```python
from build123d import *

# Parameters (mm, degrees)
SKETCH5_R               = 9.525
BOSS_EXTRUDE1_DEPTH     = 15.24
SKETCH6_R               = 12.7
BOSS_EXTRUDE2_DEPTH     = 2.54
CUT_EXTRUDE1_DEPTH      = 26.272680903
CUT_EXTRUDE3_DEPTH      = 26.272680903
CUT_EXTRUDE3_DEPTH_BACK = 26.272680903
SKETCH8_R               = 1.7526
CUT_EXTRUDE4_DEPTH      = 26.272680973
CUT_EXTRUDE4_DEPTH_BACK = 26.272680973
SKETCH9_R               = 1.7526


with BuildPart() as part:
    # Sketch5 → Boss-Extrude1 (new body)
    with BuildSketch(Plane.XY):
        with Locations(Location((0, 0, 0), (0, 0, 180))):
            Circle(SKETCH5_R)
    extrude(amount=BOSS_EXTRUDE1_DEPTH)

    # Sketch6 → Boss-Extrude2 (add)
    with BuildSketch(Plane.XY.offset(15.24)):
        Circle(SKETCH6_R)
    extrude(amount=BOSS_EXTRUDE2_DEPTH)

    # Sketch7 → Cut-Extrude1 (cut, through all)
    with BuildSketch(Plane(origin=(0, 0, 0), x_dir=(-1, 0, 0), z_dir=(0, 0, -1))):
        with BuildLine():
            ThreePointArc((4.181770846, 5.456960429), (3.437499983, 5.953924622), (2.634980936, 6.35))
            Line((2.634980936, 6.35), (-2.634980936, 6.35))
            ThreePointArc((-2.634980936, 6.35), (-3.437499983, 5.953924622), (-4.181770846, 5.456960429))
            Line((-4.181770846, 5.456960429), (-6.816751782, 0.893039571))
            ThreePointArc((-6.816751782, 0.893039571), (-6.874999966, 0), (-6.816751782, -0.893039571))
            Line((-6.816751782, -0.893039571), (-4.181770846, -5.456960429))
            ThreePointArc((-4.181770846, -5.456960429), (-3.437499983, -5.953924622), (-2.634980936, -6.35))
            Line((-2.634980936, -6.35), (2.634980936, -6.35))
            ThreePointArc((2.634980936, -6.35), (3.437499983, -5.953924622), (4.181770846, -5.456960429))
            Line((4.181770846, -5.456960429), (6.816751782, -0.893039571))
            ThreePointArc((6.816751782, -0.893039571), (6.860422465, -0.447468582), (6.874999966, 0))
            ThreePointArc((6.874999966, 0), (6.860422465, 0.447468582), (6.816751782, 0.893039571))
            Line((6.816751782, 0.893039571), (4.181770846, 5.456960429))
        make_face()
    extrude(amount=-CUT_EXTRUDE1_DEPTH, mode=Mode.SUBTRACT)

    # Sketch8 → Cut-Extrude3 (cut, two sides: drawn at the far end of the back side and taken through both)
    with BuildSketch(Plane(origin=(0, 0, 0), x_dir=(0, 0, -1), z_dir=(1, 0, 0)).offset(-CUT_EXTRUDE3_DEPTH_BACK)):
        with Locations((-8.89, 0)):
            Circle(SKETCH8_R)
    extrude(amount=CUT_EXTRUDE3_DEPTH + CUT_EXTRUDE3_DEPTH_BACK, mode=Mode.SUBTRACT)

    # Sketch9 → Cut-Extrude4 (cut, two sides: drawn at the far end of the back side and taken through both)
    with BuildSketch(Plane(origin=(0, 0, 0), x_dir=(1, 0, 0), z_dir=(0, 1, 0)).offset(-CUT_EXTRUDE4_DEPTH_BACK)):
        with Locations(Location((0, -8.89, 0), (0, 0, 270))):
            Circle(SKETCH9_R)
    extrude(amount=CUT_EXTRUDE4_DEPTH + CUT_EXTRUDE4_DEPTH_BACK, mode=Mode.SUBTRACT)


solid = part.part
```
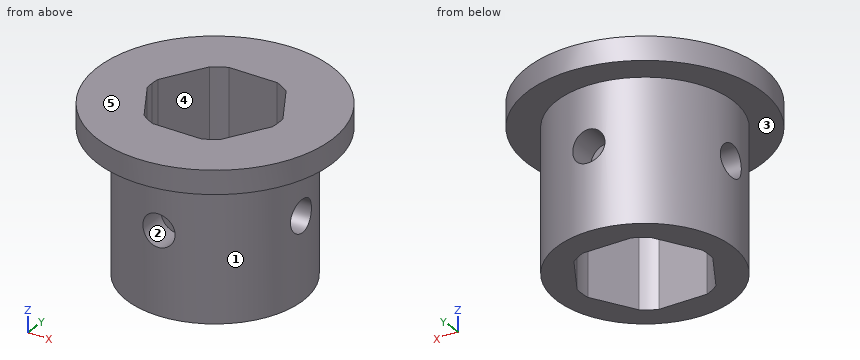
Geometry: final body of the model. Coordinates: model frame, mm. Face numbers are marked on the shaded views. A direction names the side the tool comes from. Round coordinates to 2 decimals unless told otherwise and drop trailing zeros. Order: outer loops, then holes, each group sorted by start corner. A loop starts at its lowest first (then second) coordinate and runs counter-clockwise, first axis right, second up. Notation, with made-up numbers: M 76.25,50.25 L 118.25,50.25 A25 cw 118.25,67.25 Z; hole C -23,45 d2. An arc over 180 degrees is marked long. Use one line per item in the form item = value. Start each with the question number.
Q1. Cut plane D-D (z = 5.25). Return loops of the section in (x, y) (3 decimals), and give its area (3 significant figures).
Q2. Access query for the marked faces 4 and 5. Directions: +Z, -Z, +X, -X, +Y, -Y. A direction counts if a zero-diameter tool reaches every point of the face in a straight line with its end or side. Return the directions, or none.
Q3. Material intervals for line 1 (Z direction, x = 0, y = -7.15); line 2 (X direction, y = -5.25, z = 11); line 3 (Z direction, x = 1.25, y = 10), sorted ascending. Write a range as [from, to].
Q4. Mould query, pull axis X, two halves, no side actions, for the marked faces 1, 2 and 3. Classes: +X half, -X half, draft (parallel to the pull), parting line (faces both ways), or undercut.
Q5. Cut plane A-A (x = 0). Return loops of the section in (y, z) (3 decimals), and give its area (3 significant figures).
Q6. Cut plane B-B (z = 8.89). Return loops of the section in (x, y) (3 decimals).
Q7. Cut plane C-C (y = -3). Return loops of the section in (x, z), and give its area (3 significant figures).
Q8. Pin query (flat end, axial travel): pin 1 Ø2.5 at (x, z) = (-1, 10) entering from +Y (3 decimals); pin 2 Ø6 at (y, z) = (0, 6) entering from +X (3 decimals); pin 3 Ø6 at (x, y) = (-2.5, 0) entering from -Z; pin 4 Ø4 at (x, z) = (6, 15.5) entering from +Y. Return the tip coordinate at first contact, or that it passes through.
Geometry results:
q1.outline = C 0,0 d19.05; hole M -6.817,-0.893 L -4.182,-5.457 A6.875 ccw -2.635,-6.35 L 2.635,-6.35 A6.875 ccw 4.182,-5.457 L 6.817,-0.893 A6.875 ccw 6.817,0.893 L 4.182,5.457 A6.875 ccw 2.635,6.35 L -2.635,6.35 A6.875 ccw -4.182,5.457 L -6.817,0.893 A6.875 ccw Z
q1.area = 148 mm^2
q2.face_4 = +Z, -Z
q2.face_5 = +Z, +X, -X, +Y, -Y
q3.line_1 = [0, 7.14], [10.64, 17.78]
q3.line_2 = [-7.95, -4.3], [4.3, 7.95]
q3.line_3 = [15.24, 17.78]
q4.face_1 = parting line
q4.face_2 = undercut
q4.face_3 = draft
q5.outline = M -12.7,15.24 L -9.525,15.24 L -9.525,10.643 L -6.35,10.643 L -6.35,17.78 L -12.7,17.78 Z; M -9.525,0 L -6.35,0 L -6.35,7.137 L -9.525,7.137 Z; M 6.35,0 L 9.525,0 L 9.525,7.137 L 6.35,7.137 Z; M 6.35,10.643 L 9.525,10.643 L 9.525,15.24 L 12.7,15.24 L 12.7,17.78 L 6.35,17.78 Z
q5.area = 107 mm^2
q6.outline = M -9.362,-1.753 A9.525 ccw -1.753,-9.362 L -1.753,-6.35 L -2.635,-6.35 A6.875 cw -4.182,-5.457 L -6.32,-1.753 Z; M -9.362,1.753 L -6.32,1.753 L -4.182,5.457 A6.875 cw -2.635,6.35 L -1.753,6.35 L -1.753,9.362 A9.525 ccw Z; M 1.753,-9.362 A9.525 ccw 9.362,-1.753 L 6.32,-1.753 L 4.182,-5.457 A6.875 cw 2.635,-6.35 L 1.753,-6.35 Z; M 1.753,6.35 L 2.635,6.35 A6.875 cw 4.182,5.457 L 6.32,1.753 L 9.362,1.753 A9.525 ccw 1.753,9.362 Z
q7.outline = M -12.34,15.24 L -9.04,15.24 L -9.04,0 L -5.6,0 L -5.6,17.78 L -12.34,17.78 Z; M 5.6,0 L 9.04,0 L 9.04,15.24 L 12.34,15.24 L 12.34,17.78 L 5.6,17.78 Z
q7.area = 139 mm^2
q8.pin_1 = 9.525
q8.pin_2 = 9.525
q8.pin_3 = through
q8.pin_4 = 12.05
